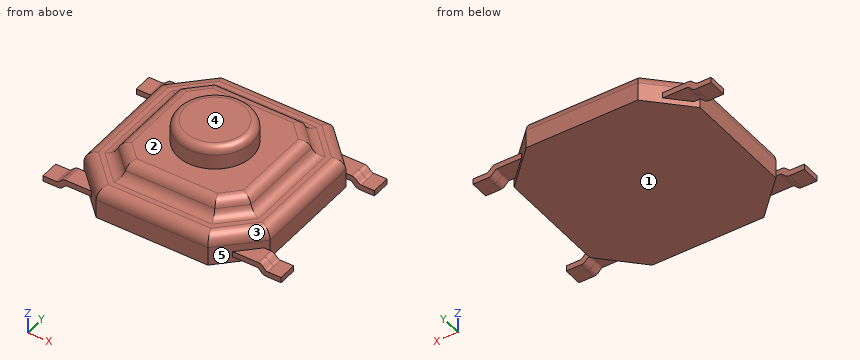
from build123d import *

# Parameters (mm, degrees)
BOSS_EXTRUDE1_DEPTH = 0.8
BOSS_EXTRUDE2_DEPTH = 0.4
SKETCH3_R           = 1
BOSS_EXTRUDE3_DEPTH = 0.6
FILLET1_R           = 0.3
FILLET2_R           = 0.3
FILLET3_R           = 0.3
FILLET4_R           = 0.2
BOSS_EXTRUDE4_DEPTH = 0.25


with BuildPart() as part:
    # Sketch1 → Boss-Extrude1 (new body)
    with BuildSketch(Plane.XY):
        Polygon((-1.5, 2.5), (1.5, 2.5), (2.5, 1.5), (2.5, -1.5), (1.5, -2.5), (-1.5, -2.5), (-2.5, -1.5), (-2.5, 1.5), align=None)
    extrude(amount=BOSS_EXTRUDE1_DEPTH)

    # Sketch2 → Boss-Extrude2 (add)
    with BuildSketch(Plane.XY.offset(0.8)):
        Polygon((-1.210050506, 1.8), (-1.8, 1.210050506), (-1.8, -1.210050506), (-1.210050506, -1.8), (1.210050506, -1.8), (1.8, -1.210050506), (1.8, 1.210050506), (1.210050506, 1.8), align=None)
    extrude(amount=BOSS_EXTRUDE2_DEPTH)

    # Sketch3 → Boss-Extrude3 (add)
    with BuildSketch(Plane.XY.offset(1.2)):
        Circle(SKETCH3_R)
    extrude(amount=BOSS_EXTRUDE3_DEPTH)

    # Fillet1
    fillet1_edges = [part.edges().sort_by_distance(p)[0] for p in [
        (1.505025253, 1.505025253, 1.2),
        (0, 1.8, 1.2),
        (-1.505025253, 1.505025253, 1.2),
        (-1.8, 0, 1.2),
        (-1.505025253, -1.505025253, 1.2),
        (0, -1.8, 1.2),
        (1.505025253, -1.505025253, 1.2),
        (1.8, 0, 1.2),
    ]]
    fillet(fillet1_edges, radius=FILLET1_R)

    # Fillet2
    fillet2_edges = [part.edges().sort_by_distance(p)[0] for p in [
        (-2, 2, 0.8),
        (-2.5, 0, 0.8),
        (-2, -2, 0.8),
        (0, -2.5, 0.8),
        (2, -2, 0.8),
        (2.5, 0, 0.8),
        (2, 2, 0.8),
        (0, 2.5, 0.8),
    ]]
    fillet(fillet2_edges, radius=FILLET2_R)

    # Fillet3
    fillet3_edges = [part.edges().sort_by_distance(p)[0] for p in [
        (0, -1.8, 0.8),
        (1.505025253, -1.505025253, 0.8),
        (1.8, 0, 0.8),
        (1.505025253, 1.505025253, 0.8),
        (0, 1.8, 0.8),
        (-1.505025253, 1.505025253, 0.8),
        (-1.8, 0, 0.8),
        (-1.505025253, -1.505025253, 0.8),
    ]]
    fillet(fillet3_edges, radius=FILLET3_R)

    # Fillet4
    fillet4_edges = [part.edges().sort_by_distance(p)[0] for p in [
        (-1, 0, 1.8),
    ]]
    fillet(fillet4_edges, radius=FILLET4_R)

    # Sketch4 → Boss-Extrude4 (add, symmetric)
    with BuildSketch(Plane(origin=(0, 1.85, 0), x_dir=(1, 0, 0), z_dir=(0, 1, 0))):
        with BuildLine():
            Line((0, -0.15), (-2.55, -0.15))
            add(Edge.make_bspline(
                [(-2.8, 0), (-2.662431202, 0), (-2.630462892, -0.15), (-2.55, -0.15)],
                knots=[0, 0, 0, 0, 1, 1, 1, 1], degree=3))
            Line((-2.8, 0), (-3.2, 0))
            Line((-3.2, 0), (-3.2, -0.15))
            Line((-3.2, -0.15), (-2.841547595, -0.15))
            add(Edge.make_bspline(
                [(-2.591547595, -0.3), (-2.713318055, -0.3), (-2.744365063, -0.15), (-2.841547595, -0.15)],
                knots=[0, 0, 0, 0, 1, 1, 1, 1], degree=3))
            Line((-2.591547595, -0.3), (0, -0.3))
            Line((0, -0.3), (2.591547595, -0.3))
            add(Edge.make_bspline(
                [(2.591547595, -0.3), (2.713318055, -0.3), (2.744365063, -0.15), (2.841547595, -0.15)],
                knots=[0, 0, 0, 0, 1, 1, 1, 1], degree=3))
            Line((2.841547595, -0.15), (3.2, -0.15))
            Line((3.2, -0.15), (3.2, 0))
            Line((3.2, 0), (2.8, 0))
            add(Edge.make_bspline(
                [(2.8, 0), (2.662431202, 0), (2.630462892, -0.15), (2.55, -0.15)],
                knots=[0, 0, 0, 0, 1, 1, 1, 1], degree=3))
            Line((2.55, -0.15), (0, -0.15))
        make_face()
    boss_extrude4 = extrude(amount=BOSS_EXTRUDE4_DEPTH, both=True)

    # Mirror1: Boss-Extrude4 across plane
    add(boss_extrude4.mirror(Plane.ZX))


solid = part.part
The listing builds one solid part. Answer for the finished solid, in the listing's coordinates (mm). Face numbers are marked on the shaded views. A direction names the side the tool comes from. Coordinates: 2 decimals unless noted, no trailing zeros. Order: outer loops, then holes, each group sorted by start corner. A loop starts at its lowest first (then second) coordinate and runs counter-clockwise, first axis right, second up. Notation, with made-up numbers: (-32, -36.5) -> (-6, -36.5) arc R34 ccw to (-6, -0.5) -> close; hole circle Ø10 at (-15, -18). An arc over 180 degrees is marked (long way). Answer in a Markdown table with one row per item. Add a question column.
Item 1: Find the intervals of material crossed by L1, parallel to Z at x = -1.25, y = 0.9; L2, parallel to X at y = 0.4, z = 0.45; L3, parallel to X at y = 0.05, z = 1.3, in increasing order. Write a range as from..to.
Item 2: Find section B-B (z = 0.7). Write down the section's boundary in (x, y), then the cut area to 3 significant figures.
Item 3: Each of these flat-tipped pins is pushed along its axis until it touches: P1, Ø0.6, axis at x = -2.5, y = -1.5, coming from the -Z side; P2, Ø1, axis at x = 0, z = 1.5, coming from the +Y side; P3, Ø0.6, axis at x = 2.5, y = 2, coming from the +Z side. Where does it stop, or does it pass through?
Item 4: Which of the six approach directions +Z, -Z, +X, -X, +Y, -Y give full straight-line access (tool end or side, diameter ignored) to the marked faces 1 and 2?
Item 5: Determine the mould class of the marked faces 3, 4 and 5 for opening direction X: +X half, -X half, draft (parallel to the pull), parting line (faces both ways), or undercut.
Item 6: Find section C-C (z = 1.5). Write down the section's boundary in (x, y), then the cut area to 3 significant figures.
Item 7: Find section A-A (z = 0.4). Write down the section's boundary in (x, y).
Result set:
| question | item | result |
|---|---|---|
| 1 | L1 | z = 0..1.2 |
| 1 | L2 | x = -2.5..2.5 |
| 1 | L3 | x = -1..1 |
| 2 | outline | (-2.42, -1.47) -> (-1.47, -2.42) -> (1.47, -2.42) -> (2.42, -1.47) -> (2.42, 1.47) -> (1.47, 2.42) -> (-1.47, 2.42) -> (-2.42, 1.47) -> close |
| 2 | area | 21.7 mm² |
| 3 | P1 | stops at z = 0 |
| 3 | P2 | stops at y = 1.78 |
| 3 | P3 | stops at z = 0.3 |
| 4 | face 1 | -Z, +X, -X, +Y, -Y |
| 4 | face 2 | +Z |
| 5 | face 3 | +X half |
| 5 | face 4 | draft |
| 5 | face 5 | undercut |
| 6 | outline | circle Ø2 at (0, 0) |
| 6 | area | 3.14 mm² |
| 7 | outline | (-2.5, -1.5) -> (-1.5, -2.5) -> (1.5, -2.5) -> (2.5, -1.5) -> (2.5, 1.5) -> (1.5, 2.5) -> (-1.5, 2.5) -> (-2.5, 1.5) -> close |
